Build history of the part. All positions in model axes, mm. Face numbers are marked on the shaded views. A direction names the side the tool comes from. Give positions to 0.01 mm unless a question says otherwise; leave off trailing zeros. Order: outer loops, then holes, each group sorted by start corner. A loop starts at its lowest first (then second) coordinate and runs counter-clockwise, first axis right, second up. Notation, with made-up numbers: (89.25, 20) - (94.25, 20) arc R22 cw to (94.25, 44) - close; hole circle Ø8 at (4, 20.25). An arc over 180 degrees is marked (long way). Answer in a Markdown table with one row per item.
```python
from build123d import *


with BuildPart() as part:
    # Croquis1 → Revolución1 (revolve)
    with BuildSketch(Plane(origin=(0, 0, 0), x_dir=(0, 0, -1), z_dir=(1, 0, 0)), mode=Mode.PRIVATE) as revoluci_n1_sk:
        Polygon((13.7, 0), (-41.3, 0), (-41.3, 3), (0, 3), (0, 10), (-6, 10), (-6, 15), (-2, 15), (-2, 27), (-1, 27), (-1, 30), (-2, 30), (-2, 31), (11, 31), (11, 29), (3, 29), (3, 22), (6, 22), (6, 14), (5, 14), (5, 9), (10, 9), (10, 3), (13.7, 3), align=None)
    revolve(revoluci_n1_sk.sketch.rotate(Axis((0, 0, -13.7), (0, 0, 1)), 90), axis=Axis((0, 0, -13.7), (0, 0, 1)))


solid = part.part
```
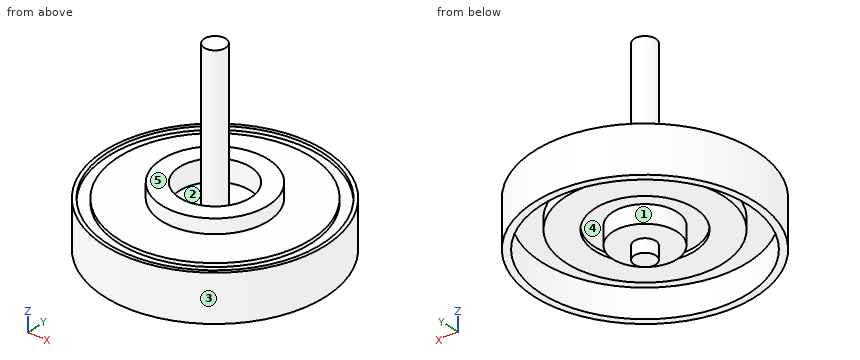
1. Cut at C-C on z = -2. Write the cut outline in (x, y).
Check result:
| item | result |
|---|---|
| outline | circle Ø62 at (0, 0) |
2. Drop flat-ended pins along their axis: P1, Ø6, axis at x = -24, y = -11.5, coming from the +Z side; P2, Ø17.5, axis at x = 5.5, y = -4, coming from the -Z side; P3, Ø2, axis at x = 4, z = -1, coming from the -Y side; P4, Ø6, axis at y = -3, z = 18.5, coming from the -X side. Give the stop position or say it passes through.
Check result:
| item | result |
|---|---|
| P1 | stops at z = 2 |
| P2 | stops at z = -13.7 |
| P3 | stops at y = -30.85 |
| P4 | stops at x = -3 |
3. Cut at A-A on y = 17.5. Write the cut outline in (x, z).
Check result:
| item | result |
|---|---|
| outline | (-25.59, -11) - (-23.12, -11) - (-23.12, -3) - (-13.33, -3) - (-13.33, -6) - (13.33, -6) - (13.33, -3) - (23.12, -3) - (23.12, -11) - (25.59, -11) - (25.59, 2) - (24.37, 2) - (24.37, 1) - (20.56, 1) - (20.56, 2) - (-20.56, 2) - (-20.56, 1) - (-24.37, 1) - (-24.37, 2) - (-25.59, 2) - close |
4. Cut at B-B on x = 16.5. Write the cut outline in (y, z), and give its area (3 significant figures).
Check result:
| item | result |
|---|---|
| outline | (-26.24, -11) - (-23.85, -11) - (-23.85, -3) - (-14.55, -3) - (-14.55, -6) - (14.55, -6) - (14.55, -3) - (23.85, -3) - (23.85, -11) - (26.24, -11) - (26.24, 2) - (25.05, 2) - (25.05, 1) - (21.37, 1) - (21.37, 2) - (-21.37, 2) - (-21.37, 1) - (-25.05, 1) - (-25.05, 2) - (-26.24, 2) - close |
| area | 381 mm² |
5. Probe line 1 (Y direction, x = 0, z = 1.45); line 2 (Y direction, x = 0, z = -7.5); line 3 (Y direction, x = 0, z = -4.75). List the from-to ranges inside material, lowest first.
Check result:
| item | result |
|---|---|
| line 1 | y = -31 to -30, -27 to -10, -3 to 3, 10 to 27, 30 to 31 |
| line 2 | y = -31 to -29, -9 to 9, 29 to 31 |
| line 3 | y = -31 to -29, -22 to 22, 29 to 31 |
6. Two-plate mould, pull along X, no slides. Class the marked faces 3, 4 and 5: +X half, -X half, draft (parallel to the pull), parting line (faces both ways), or undercut.
Check result:
| item | result |
|---|---|
| face 3 | parting line |
| face 4 | undercut |
| face 5 | draft |
7. Cut at D-D on x = -26. Write the cut outline in (y, z), and give its area (3 significant figures).
Check result:
| item | result |
|---|---|
| outline | (-16.88, -11) - (-12.85, -11) - (-12.85, -3) - (12.85, -3) - (12.85, -11) - (16.88, -11) - (16.88, 2) - (14.97, 2) - (14.97, 1) - (7.28, 1) - (7.28, 2) - (-7.28, 2) - (-7.28, 1) - (-14.97, 1) - (-14.97, 2) - (-16.88, 2) - close |
| area | 218 mm² |
8. Which spindle directions (+Z, -Z, +X, -X, +Y, -Y) get a long thin tool onto all of the face, cutting with end or side? Do the marked faces 1 and 2. Say none if no direction does.
Check result:
| item | result |
|---|---|
| face 1 | -Z |
| face 2 | +Z |
